```python
from build123d import *

# Parameters (mm, degrees)
SKETCH2_R                = 2.5
BOSS_EXTRUDE1_DEPTH      = 100
BOSS_EXTRUDE2_DEPTH      = 200
CUT_EXTRUDE5_START       = 60.350129398
CUT_EXTRUDE5_DEPTH       = 39.299741204
CIRPATTERN2_COUNT        = 2
CUT_EXTRUDE13_START      = 60.350129398
CUT_EXTRUDE13_DEPTH      = 39.299741204
FILLET1_R                = 10
FILLET2_R                = 10
CUT_EXTRUDE14_DEPTH      = 105.432992871
CUT_EXTRUDE14_DEPTH_BACK = 105.432992871
SKETCH14_W               = 44.068346903
SKETCH14_H               = 27.8913588
CUT_EXTRUDE15_DEPTH      = 91.768685539
CUT_EXTRUDE15_DEPTH_BACK = 91.768685539
SKETCH15_W               = 22.136968411
SKETCH15_H               = 5.24183176
CUT_EXTRUDE16_DEPTH      = 89.750452329
CUT_EXTRUDE16_DEPTH_BACK = 89.750452329
SKETCH16_W               = 11.028183549
SKETCH16_H               = 76.248198314
CUT_EXTRUDE17_DEPTH      = 89.750452329
CUT_EXTRUDE17_DEPTH_BACK = 89.750452329
SKETCH19_W               = 10.280501296
SKETCH19_H               = 4.008748932
SKETCH20_R               = 0.5
BOSS_EXTRUDE3_DEPTH      = 7.5


# Read off the part's stored shape, not the designer's step: Cut-Extrude5, Cut-Extrude13
with BuildPart() as part:
    # Sketch2 → Boss-Extrude1 (new body)
    with BuildSketch(Plane(origin=(0, 0, 0), x_dir=(1, 0, 0), z_dir=(0, 1, 0))):
        with Locations(Location((0, 0, 0), (0, 0, 270))):
            Circle(SKETCH2_R)
    extrude(amount=BOSS_EXTRUDE1_DEPTH)

    # Sketch3 → Boss-Extrude2 (add)
    with BuildSketch(Plane.XY):
        Polygon((47.096645081, 63.143071984), (-46.001441122, 99.649870602), (-47.096645081, 96.856928016), (46.001441122, 60.350129398), align=None)
    boss_extrude2 = extrude(amount=-BOSS_EXTRUDE2_DEPTH)

    # Cut-Extrude5 outline → Cut-Extrude5 (cut)
    with BuildSketch(Plane(origin=(0, 0, 0), x_dir=(1, 0, 0), z_dir=(0, 1, 0)).offset(CUT_EXTRUDE5_START)):
        Polygon((-2.5, 0), (-2.5, 30), (2.5, 30), (2.5, 0), (49, 0), (49, 200), (-49, 200), (-49, 0), align=None)
    extrude(amount=CUT_EXTRUDE5_DEPTH, mode=Mode.SUBTRACT)

    # CirPattern2: Boss-Extrude2 ×2 about axis
    cirpattern2_axis = Axis((0, 100, 0), (0, -1, 0))
    for i in range(1, CIRPATTERN2_COUNT):
        add(boss_extrude2.rotate(cirpattern2_axis, i * 360 / CIRPATTERN2_COUNT))

    # Cut-Extrude13 outline → Cut-Extrude13 (cut)
    with BuildSketch(Plane(origin=(0, 0, 0), x_dir=(1, 0, 0), z_dir=(0, 1, 0)).offset(CUT_EXTRUDE13_START)):
        Polygon((-2.5, -30), (-2.5, 0), (-49, 0), (-49, -200), (49, -200), (49, 0), (2.5, 0), (2.5, -30), align=None)
    extrude(amount=CUT_EXTRUDE13_DEPTH, mode=Mode.SUBTRACT)

    # Fillet1
    # the kernel refuses this fillet: 10 mm, written as the material it takes off along each edge
    with BuildSketch(Plane(origin=(2.5, 55.757829393, -30), x_dir=(0, 0, 1), z_dir=(0, 1, 0))) as fillet1_piece_1:
        with BuildLine():
            CenterArc((8.660254038, -10), FILLET1_R, 90, 60)
            Line((0, -5), (-0.173205081, -4.9))
            ThreePointArc((-0.173205081, -4.9), (-0.2, -2.5), (-0.2, 0))
            Line((-0.2, 0), (0, 0.2))
            Line((0, 0.2), (8.660254038, 0.2))
            Line((8.660254038, 0.2), (8.660254038, 0))
        make_face()
    extrude(amount=46.523677998, mode=Mode.SUBTRACT)

    # Fillet2
    # the kernel refuses this fillet: 10 mm, written as the material it takes off along each edge
    with BuildSketch(Plane(origin=(-2.5, 55.757829393, 30), x_dir=(0, 0, -1), z_dir=(0, 1, 0))) as fillet2_piece_1:
        with BuildLine():
            CenterArc((8.660254038, -10), FILLET2_R, 90, 60)
            Line((0, -5), (-0.173205081, -4.9))
            ThreePointArc((-0.173205081, -4.9), (-0.2, -2.5), (-0.2, 0))
            Line((-0.2, 0), (0, 0.2))
            Line((0, 0.2), (8.660254038, 0.2))
            Line((8.660254038, 0.2), (8.660254038, 0))
        make_face()
    extrude(amount=46.523677998, mode=Mode.SUBTRACT)

    # Sketch14 → Cut-Extrude14 (cut, two sides: drawn at the far end of the back side and taken through both)
    with BuildSketch(Plane(origin=(0, 0, 0), x_dir=(0, 0, -1), z_dir=(1, 0, 0)).offset(-CUT_EXTRUDE14_DEPTH_BACK)):
        with Locations((-11.714370696, 99.576890266)):
            Rectangle(SKETCH14_W, SKETCH14_H)
    extrude(amount=CUT_EXTRUDE14_DEPTH + CUT_EXTRUDE14_DEPTH_BACK, mode=Mode.SUBTRACT)

    # Sketch15 → Cut-Extrude15 (cut, two sides: drawn at the far end of the back side and taken through both)
    with BuildSketch(Plane(origin=(0, 0, 0), x_dir=(0, 0, -1), z_dir=(1, 0, 0)).offset(-CUT_EXTRUDE15_DEPTH_BACK)):
        with Locations((-5.158121646, 86.109794113)):
            Rectangle(SKETCH15_W, SKETCH15_H)
    extrude(amount=CUT_EXTRUDE15_DEPTH + CUT_EXTRUDE15_DEPTH_BACK, mode=Mode.SUBTRACT)

    # Sketch16 → Cut-Extrude16 (cut, two sides: drawn at the far end of the back side and taken through both)
    with BuildSketch(Plane(origin=(0, 0, 0), x_dir=(0, 0, -1), z_dir=(1, 0, 0)).offset(-CUT_EXTRUDE16_DEPTH_BACK)):
        with Locations((1.378247022, 35.930712441)):
            Rectangle(SKETCH16_W, SKETCH16_H)
    extrude(amount=CUT_EXTRUDE16_DEPTH + CUT_EXTRUDE16_DEPTH_BACK, mode=Mode.SUBTRACT)

    # Sketch19 → Cut-Extrude17 (cut, two sides: drawn at the far end of the back side and taken through both)
    with BuildSketch(Plane(origin=(0, 0, 0), x_dir=(0, 0, -1), z_dir=(1, 0, 0)).offset(-CUT_EXTRUDE17_DEPTH_BACK)):
        with Locations((0.096985861, 73.82556599)):
            Rectangle(SKETCH19_W, SKETCH19_H)
    extrude(amount=CUT_EXTRUDE17_DEPTH + CUT_EXTRUDE17_DEPTH_BACK, mode=Mode.SUBTRACT)

    # Sketch20 → Boss-Extrude3 (add)
    with BuildSketch(Plane.XZ.offset(-75.829940456)):
        with Locations(Location((0, 0, 0), (0, 0, 270))):
            Circle(SKETCH20_R)
    extrude(amount=BOSS_EXTRUDE3_DEPTH)


solid = part.part
```
Verification items for the finished model (mm, model axes). A direction names the side the tool comes from. Round coordinates to 2 decimals unless told otherwise and drop trailing zeros. Loops run counter-clockwise (first coordinate to the right, second up) from the corner with the lowest first, then second, coordinate; pieces in that order, holes last. Notation, with made-up numbers: (-14, 22) -> (26, 22) arc R19 ccw to (26, 53) -> close; hole circle Ø1 at (70, -9). An arc over 180 degrees is marked (long way). Answer as a JSON object with one key per item and string values.
Q1. Section check D-D (z = 25.5). Record the boundary of the cut face in (x, y), then the cut area to 3 significant figures.
Data:
{"outline": "(-1.59, 77.76) -> (2.5, 79.37) -> (2.5, 82.59) -> (-1.59, 80.99) -> close", "area": "13.2 mm2"}
Q2. Scan lines: line 1 (Z direction, x = 0.2, y = 77.5); line 2 (Y direction, x = -0.9, z = 15); line 3 (Y direction, x = 2.2, z = -15). Record each from-to range of solid material in increasing order. Write a range as from..to.
Data:
{"line 1": "z = -2.49..2.49", "line 2": "y = 78.04..81.26", "line 3": "y = 77.53..80.75"}
Q3. Section check A-A (y = 70.25). Record the boundary of the cut face in (x, z), then the cut area to 3 significant figures.
Data:
{"outline": "circle Ø1 at (0, 0)", "area": "0.785 mm2"}
Q4. Access from +Z, -Z, +X, -X, +Y, -Y to the whole of each face (thin tool, end or side, straight path). Record for faces 4 (the cylindrical face through (-1.197, 79.964, 26.276)), 5 (the cylindrical face through (-2.22, 77.18, 1.15)).
Data:
{"face 4": "+Z, -X, +Y, -Y", "face 5": "-Y"}
Q5. Draft check along Y on faces 1 (the flat face through (-2.5, 80, -4)), 2 (the flat face through (0.035, 78.403, 14.79)), 3 (the flat face through (-0.035, 81.597, 14.79)). Enter one of: pulls with the +Y half, pulls with the -Y half, needs draft (parallel to the pull), parting line crosses it, or undercut.
Data:
{"face 1": "needs draft", "face 2": "pulls with the -Y half", "face 3": "pulls with the +Y half"}
Q6. Section check C-C (z = -9). Record the boundary of the cut face in (x, y).
Data:
{"outline": "(-2.5, 79.37) -> (2.5, 77.41) -> (2.5, 80.63) -> (-2.5, 82.59) -> close"}
Q7. Section check B-B (x = -1.8). Record the boundary of the cut face in (y, z).
Data:
{"outline": "(75.83, -1.73) -> (79.09, -1.73) -> (79.09, -29.56) -> (82.32, -29.56) -> (82.32, -1.73) -> (83.49, -1.73) -> (83.49, 1.73) -> (80.91, 1.73) -> (80.91, 25.02) -> (77.68, 25.02) -> (77.68, 1.73) -> (75.83, 1.73) -> close"}
Q8. Go/stop test with flat-tipped pins: P1, Ø1.5, axis at x = 0, z = 9, coming from the +Y side; P2, Ø5, axis at y = 73, z = -1, coming from the +X side. Record where each tip stops, or that it passes through.
Data:
{"P1": "stops at y = 81.91", "P2": "stops at x = 0.5"}
